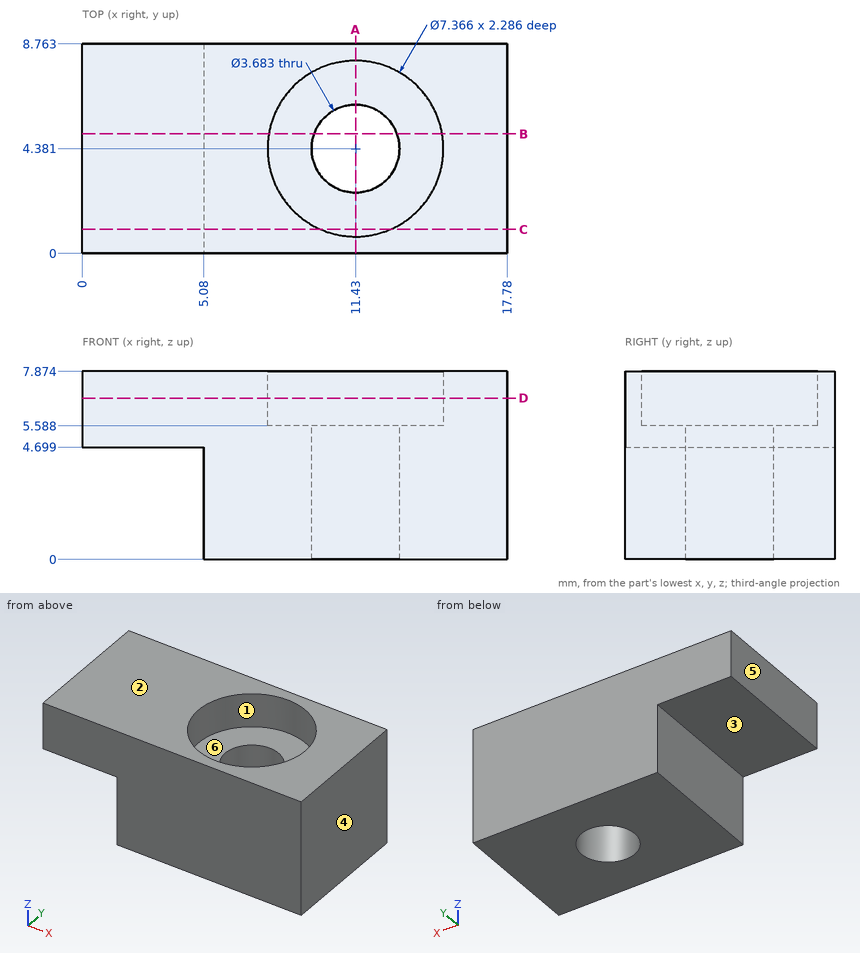
For this review, use the dimensioned drawing (mm, ordinates from the lowest corner) and the shaded views. A direction names the side the tool comes from. Round coordinates to 2 decimals unless told otherwise and drop trailing zeros. Write each loop counter-clockwise with the first axis right and the second up, starting at its lowest first coordinate (ties: lowest second). Pieces come first, ordered by that corner, then holes. Notation, with made-up numbers: (18, 56) -> (76, 56) arc R13 ccw to (76, 65) -> close; hole circle Ø7 at (-38, 21). An arc over 180 degrees is marked (long way). Answer in a Markdown table with one row per item.
Q1. To check wall thickness, follow L1, parallel to Y at x = 11.43, z = 7.2 (1 decimal); L2, parallel to X at y = 2.5, z = 4; L3, parallel to Y at x = 13.5, z = 7.75 (1 decimal). State the ranges of each line that lie inside material, in increasing order. Write a range as [from, to].
The answers:
| item | result |
|---|---|
| L1 | [0, 0.7], [8.1, 8.8] |
| L2 | [5.08, 17.78] |
| L3 | [0, 1.3], [7.4, 8.8] |
Q2. For the marked faces 1, 2 and 3, list the 3-axis set-ups (+Z, -Z, +X, -X, +Y, -Y) from which the entire face can be reached by the end or side of a thin tool; tool diameter is ignored.
The answers:
| item | result |
|---|---|
| face 1 | +Z |
| face 2 | +Z, +X, -X, +Y, -Y |
| face 3 | -Z, -X, +Y, -Y |
Q3. Draft analysis for pull direction X (two halves, no side actions). For the marked faces 4, 5 and 6, state which applies: +X half, -X half, draft (parallel to the pull), parting line (faces both ways), or undercut.
The answers:
| item | result |
|---|---|
| face 4 | +X half |
| face 5 | -X half |
| face 6 | undercut |
Q4. Clearance check with flat-ended pins moving along their axes: pin 1 Ø2 at (y, z) = (6.5, 3.5) entering from -X; pin 2 Ø4 at (x, y) = (2, 5) entering from -Z. State where each tip first meets the part, or that it passes through.
The answers:
| item | result |
|---|---|
| pin 1 | x = 5.08 |
| pin 2 | z = 4.7 |
Q5. Take a section at B-B, the plane y = 5. State the section outline as (x, z) points (1 decimal).
The answers:
| item | result |
|---|---|
| outline | (0, 4.7) -> (5.1, 4.7) -> (5.1, 0) -> (9.7, 0) -> (9.7, 5.6) -> (7.8, 5.6) -> (7.8, 7.9) -> (0, 7.9) -> close; (13.2, 0) -> (17.8, 0) -> (17.8, 7.9) -> (15.1, 7.9) -> (15.1, 5.6) -> (13.2, 5.6) -> close |
Q6. Take a section at D-D, the plane z = 6.75. State the section outline as (x, y) points (1 decimal), then the cut area to 3 significant figures.
The answers:
| item | result |
|---|---|
| outline | (0, 0) -> (17.8, 0) -> (17.8, 8.8) -> (0, 8.8) -> close; hole circle Ø7.4 at (11.4, 4.4) |
| area | 113 mm² |
Q7. Take a section at A-A, the plane x = 11.43. State the section outline as (y, z) points (1 decimal).
The answers:
| item | result |
|---|---|
| outline | (0, 0) -> (2.5, 0) -> (2.5, 5.6) -> (0.7, 5.6) -> (0.7, 7.9) -> (0, 7.9) -> close; (6.2, 0) -> (8.8, 0) -> (8.8, 7.9) -> (8.1, 7.9) -> (8.1, 5.6) -> (6.2, 5.6) -> close |
Q8. Take a section at C-C, the plane y = 1. State the section outline as (x, z) points (1 decimal).
The answers:
| item | result |
|---|---|
| outline | (0, 4.7) -> (5.1, 4.7) -> (5.1, 0) -> (17.8, 0) -> (17.8, 7.9) -> (12.9, 7.9) -> (12.9, 5.6) -> (10, 5.6) -> (10, 7.9) -> (0, 7.9) -> close |
